Read the model definition and answer for the solid it produces. Units are mm, in the model's axes. Give positions to 0.01 mm unless a question says otherwise; leave off trailing zeros. Loops run counter-clockwise (first coordinate to the right, second up) from the corner with the lowest first, then second, coordinate; pieces in that order, holes last. Notation, with made-up numbers: (75.5, 61) -> (134.5, 61) arc R24 ccw to (134.5, 85) -> close; hole circle Ø9 at (-23.75, -5.5). An arc over 180 degrees is marked (long way). Write each question's results on one line, items separated by ' | '. Start each with the question number.
Item 1: Find the intervals of material crossed by line 1 (Y direction, x = 865.5, z = 6); line 2 (X direction, y = -35.5, z = -6.5); line 3 (Z direction, x = 1.6, y = -30), in increasing order.
Item 2: Each of these flat-tipped pins is pushed along its axis until it touches: P1, Ø3, axis at x = 318, z = -4, coming from the -Y side; P2, Ø4, axis at x = 515, z = -7.5, coming from the +Y side; P3, Ø5, axis at y = 30, z = 0, coming from the -X side. Where does it stop, or does it pass through?
Item 3: Section A-A on x = 1210 is taken. Write down the section's boundary in (y, z).
```python
from build123d import *

# Parameters (mm, degrees)
F2_DEPTH = 2898
F4_DEPTH = 3
F5_D     = 8
F6_R     = 4
F7_DEPTH = 3


with BuildPart() as f2:
    # F0 (on Right) → F2 (new body, through all)
    with BuildSketch(Plane.YZ):
        with BuildLine():
            Line((-12, -15), (12, -15))
            ThreePointArc((12, -15), (14.12132, -14.12132), (15, -12))
            Line((15, -12), (15, 12))
            ThreePointArc((15, 12), (14.12132, 14.12132), (12, 15))
            Line((12, 15), (-12, 15))
            ThreePointArc((-12, 15), (-14.12132, 14.12132), (-15, 12))
            Line((-15, 12), (-15, -12))
            ThreePointArc((-15, -12), (-14.12132, -14.12132), (-12, -15))
        make_face()
        with BuildLine():
            ThreePointArc((12, -10), (11.414214, -11.414214), (10, -12))
            Line((10, -12), (-10, -12))
            ThreePointArc((-10, -12), (-11.414214, -11.414214), (-12, -10))
            Line((-12, -10), (-12, 10))
            ThreePointArc((-12, 10), (-11.414214, 11.414214), (-10, 12))
            Line((-10, 12), (10, 12))
            ThreePointArc((10, 12), (11.414214, 11.414214), (12, 10))
            Line((12, 10), (12, -10))
        make_face(mode=Mode.SUBTRACT)
    extrude(amount=F2_DEPTH)

    # F3 (on Right) → F4 (join)
    with BuildSketch(Plane.YZ):
        with BuildLine():
            ThreePointArc((45, 13), (44.414214, 14.414214), (43, 15))
            Line((43, 15), (-43, 15))
            ThreePointArc((-43, 15), (-44.414214, 14.414214), (-45, 13))
            Line((-45, 13), (-45, -13))
            ThreePointArc((-45, -13), (-44.414214, -14.414214), (-43, -15))
            Line((-43, -15), (43, -15))
            ThreePointArc((43, -15), (44.414214, -14.414214), (45, -13))
            Line((45, -13), (45, 13))
        make_face()
    extrude(amount=F4_DEPTH)

    # F5 (through all)
    with Locations(Plane(origin=(0, 0, 0), x_dir=(0, 1, 0), z_dir=(-1, 0, 0))):
        with Locations((30, 0), (-30, 0)):
            Hole(F5_D / 2)

    # F6 (on offset) → F7 (join)
    with BuildSketch(Plane.YZ.offset(2898)):
        with BuildLine():
            ThreePointArc((45, 13), (44.414214, 14.414214), (43, 15))
            Line((43, 15), (-43, 15))
            ThreePointArc((-43, 15), (-44.414214, 14.414214), (-45, 13))
            Line((-45, 13), (-45, -13))
            ThreePointArc((-45, -13), (-44.414214, -14.414214), (-43, -15))
            Line((-43, -15), (43, -15))
            ThreePointArc((43, -15), (44.414214, -14.414214), (45, -13))
            Line((45, -13), (45, 13))
        make_face()
        with Locations((-30, 0)):
            Circle(F6_R, mode=Mode.SUBTRACT)
        with Locations((30, 0)):
            Circle(F6_R, mode=Mode.SUBTRACT)
    extrude(amount=-F7_DEPTH)


solid = f2.part
```
Findings:
1) line 1: -15 to -12, 12 to 15 | line 2: 0 to 3, 2895 to 2898 | line 3: -15 to -4, 4 to 15
2) P1: y = -15 | P2: y = 15 | P3: through
3) outline: (-15, -12) arc R3 ccw to (-12, -15) -> (12, -15) arc R3 ccw to (15, -12) -> (15, 12) arc R3 ccw to (12, 15) -> (-12, 15) arc R3 ccw to (-15, 12) -> close; hole (-12, -10) arc R2 ccw to (-10, -12) -> (10, -12) arc R2 ccw to (12, -10) -> (12, 10) arc R2 ccw to (10, 12) -> (-10, 12) arc R2 ccw to (-12, 10) -> close
